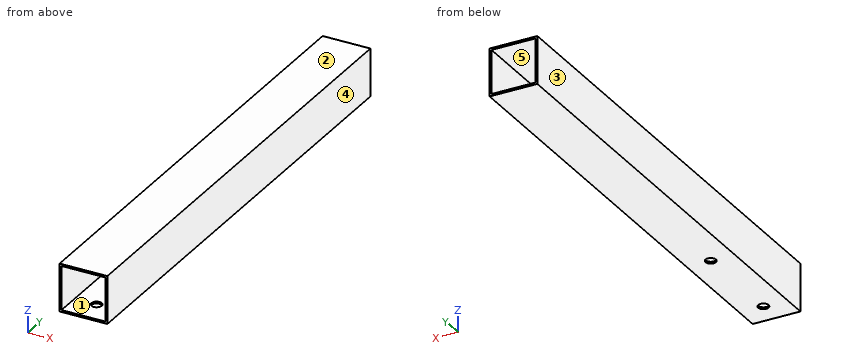
```python
from build123d import *

# Parameters (mm, degrees)
F0_W     = 50
F0_H     = 50
F0_W_2   = 46
F0_H_2   = 46
F1_DEPTH = 250
F3_D     = 11
F3_DEPTH = 2
F3_TIP   = 3.3047334047


with BuildPart() as f1:
    # F0 (on Front) → F1 (new body, symmetric)
    with BuildSketch(Plane.XZ):
        Rectangle(F0_W, F0_H)
        Rectangle(F0_W_2, F0_H_2, mode=Mode.SUBTRACT)
    extrude(amount=F1_DEPTH, both=True)

    # F3
    with Locations(Plane(origin=(0, 0, -25), x_dir=(1, 0, 0), z_dir=(0, 0, -1))):
        with Locations((0, 225), (0, 125)):
            Hole(F3_D / 2, depth=F3_DEPTH)
            with Locations((0, 0, -(F3_DEPTH + F3_TIP / 2))):  # 118° drill point
                Cone(0, F3_D / 2, F3_TIP, mode=Mode.SUBTRACT)


solid = f1.part
```
Build history of the part. All positions in model axes, mm. Face numbers are marked on the shaded views. A direction names the side the tool comes from. Coordinates: 2 decimals unless noted, no trailing zeros. Order: outer loops, then holes, each group sorted by start corner. A loop starts at its lowest first (then second) coordinate and runs counter-clockwise, first axis right, second up. Notation, with made-up numbers: M 51.25,39 L 79.25,39 A34 ccw 79.25,70 Z; hole C 89,-16.5 d10. An arc over 180 degrees is marked long. One line per question, with ' | ' between items. Start each with the question number.
1. Mould opens along Z. For the marked faces 1, 2 and 3 say: +Z half, -Z half, draft (parallel to the pull), parting line (faces both ways), or undercut.
2. Flat gauge pin, fed straight in: P1, Ø9, axis at x = 0, y = -225, coming from the -Z side. Where does the tip first touch, or does it go through?
3. Cut at B-B (z = -2). Write the cut outline in (x, y), plus the area to 3 significant figures.
4. Tool access for the marked faces 4 and 5: list every direction of +Z, -Z, +X, -X, +Y, -Y with a clear straight run to the whole face (end or side of a thin tool).
5. Wall check: line 1 along Y through (x, z) = (0, -24.15); line 2 along X through (y, z) = (-40, -14). Give the ranges that are in metal, low to high. Write a range as [from, to].
6. Cut at A-A (y = 51). Write the cut outline in (x, z), plus the area to 3 significant figures.
7. Cut at D-D (y = -125). Write the cut outline in (x, z), plus the area to 3 significant figures.
8. Cut at C-C (x = 0). Write the cut outline in (y, z), plus the area to 3 significant figures.
The answers:
1) face 1: undercut | face 2: +Z half | face 3: draft
2) P1: stops at z = 23
3) outline: M -25,-250 L -23,-250 L -23,250 L -25,250 Z; M 23,-250 L 25,-250 L 25,250 L 23,250 Z | area: 2,000 mm2
4) face 4: +Z, -Z, +X, +Y, -Y | face 5: +Y, -Y
5) line 1: y = [-250, -230.5], [-219.5, -130.5], [-119.5, 250] | line 2: x = [-25, -23], [23, 25]
6) outline: M -25,-25 L 25,-25 L 25,25 L -25,25 Z; hole M -23,-23 L 23,-23 L 23,23 L -23,23 Z | area: 384 mm2
7) outline: M -25,-25 L -5.5,-25 L -5.5,-23 L -23,-23 L -23,23 L 23,23 L 23,-23 L 5.5,-23 L 5.5,-25 L 25,-25 L 25,25 L -25,25 Z | area: 362 mm2
8) outline: M -250,-25 L -230.5,-25 L -230.5,-23 L -250,-23 Z; M -250,23 L 250,23 L 250,25 L -250,25 Z; M -219.5,-25 L -130.5,-25 L -130.5,-23 L -219.5,-23 Z; M -119.5,-25 L 250,-25 L 250,-23 L -119.5,-23 Z | area: 1,960 mm2
